Could you check a few things on this model? Use its own coordinates, in mm. Give positions to 0.01 mm unless a question says otherwise; leave off trailing zeros. Order: outer loops, then holes, each group sorted by start corner. A loop starts at its lowest first (then second) coordinate and runs counter-clockwise, first axis right, second up.
(1) Imagine slicing it at B-B, the plane y = -2.5. Write out the boundary of the cut face in (x, z), then the cut area to 3 significant figures.
(2) Will these pins go through, and if not, where does the flat tip stop? pin 1 (1.1 mm diameter, centred on x = -58, y = -57.5, fed in from +Z); pin 2 (1.2 mm diameter, centred on x = 0, y = -29, fed in from +Z); pin 3 (0.5 mm diameter, centred on x = -52.5, y = -0.5, fed in from +Z).
(3) Imagine slicing it at A-A, the plane x = -60. Write out the boundary of the cut face in (y, z), then the cut area to 3 significant figures.
(4) If I drill on probe 1 along X at (y, z) = (-3, 1.5); probe 2 along Y at (x, z) = (-51, 2.6); probe 3 along Y at (x, z) = (-28.5, 0.15), over which ranges is the centre line in solid material (lowest first)?
(5) Imagine slicing it at C-C, the plane z = 0.55. Write out the boundary of the cut face in (x, y).
(6) Imagine slicing it at D-D, the plane y = -27. Write out the boundary of the cut face in (x, z).
from build123d import *

# Parameters (mm, degrees)
F0_W     = 74
F0_H     = 64
F0_W_2   = 68
F0_H_2   = 58
F0_W_3   = 66
F0_H_3   = 56
F1_DEPTH = 2
F2_W     = 74
F2_H     = 64
F3_DEPTH = 1
F4_W     = 15
F4_H     = 6.5584733043
F4_H_2   = 3
F4_H_3   = 6.1532862581
F4_W_2   = 4
F4_H_4   = 15
F4_W_3   = 1.5584733043
F4_W_4   = 10.1532862581
F5_DEPTH = 2


with BuildPart() as f1:
    # F0 (on Top) → F1 (new body)
    with BuildSketch(Plane.XY):
        with Locations((-34, -29)):
            Rectangle(F0_W, F0_H)
        with Locations((-34, -29)):
            Rectangle(F0_W_2, F0_H_2, mode=Mode.SUBTRACT)
        with Locations((-34, -29)):
            Rectangle(F0_W_2, F0_H_2)
        with Locations((-34, -29)):
            Rectangle(F0_W_3, F0_H_3, mode=Mode.SUBTRACT)
    extrude(amount=F1_DEPTH)

    # F2 (on face) → F3 (join)
    with BuildSketch(Plane.XY.offset(2)):
        with Locations((-34, -29)):
            Rectangle(F2_W, F2_H)
        Polygon((-67, 0), (-1, 0), (-1, -1), (-1, -57), (-1, -58), (-67, -58), (-67, -57), (-67, -1), align=None, mode=Mode.SUBTRACT)
    extrude(amount=F3_DEPTH)

    # F4 (on face) → F5 (cut)
    with BuildSketch(Plane.XY.offset(3)):
        with Locations((-34, 6.2792366521)):
            Rectangle(F4_W, F4_H)
        with Locations((-34, 1.5)):
            Rectangle(F4_W, F4_H_2)
        with Locations((-34, -3.0766431291)):
            Rectangle(F4_W, F4_H_3)
        with Locations((1, -29)):
            Rectangle(F4_W_2, F4_H_4)
        with Locations((3.7792366521, -29)):
            Rectangle(F4_W_3, F4_H_4)
        with Locations((-6.0766431291, -29)):
            Rectangle(F4_W_4, F4_H_4)
        with Locations((-34, -59.5)):
            Rectangle(F4_W, F4_H_2)
        with Locations((-34, -54.9233568709)):
            Rectangle(F4_W, F4_H_3)
        with Locations((-34, -64.2792366521)):
            Rectangle(F4_W, F4_H)
        with Locations((-61.9233568709, -29)):
            Rectangle(F4_W_4, F4_H_4)
        with Locations((-69, -29)):
            Rectangle(F4_W_2, F4_H_4)
        with Locations((-71.7792366521, -29)):
            Rectangle(F4_W_3, F4_H_4)
    extrude(amount=-F5_DEPTH, mode=Mode.SUBTRACT)


solid = f1.part
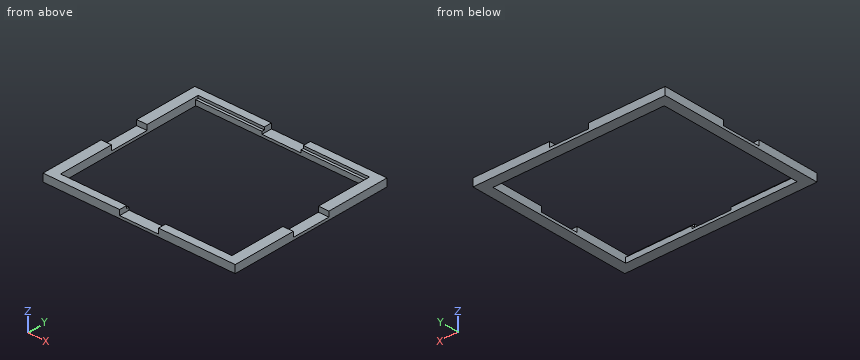
Answer block:
1. outline: (-71, 0) - (-67, 0) - (-67, 3) - (-71, 3) - close; (-1, 0) - (3, 0) - (3, 3) - (-1, 3) - close
1. area: 24.0 mm2
2. pin 1: stops at z = 3
2. pin 2: stops at z = 1
2. pin 3: stops at z = 2
3. outline: (-61, 0) - (-57, 0) - (-57, 2) - (-58, 2) - (-58, 3) - (-61, 3) - close; (-1, 0) - (3, 0) - (3, 3) - (0, 3) - (0, 2) - (-1, 2) - close
3. area: 22.0 mm2
4. probe 1: x = -71 to -67, -1 to 3
4. probe 2: y = -61 to -58, 0 to 3
4. probe 3: y = -61 to -57, -1 to 3
5. outline: (-71, -61) - (3, -61) - (3, 3) - (-71, 3) - close; hole (-67, -57) - (-1, -57) - (-1, -1) - (-67, -1) - close
6. outline: (-71, 0) - (-67, 0) - (-67, 1) - (-71, 1) - close; (-1, 0) - (3, 0) - (3, 1) - (-1, 1) - close
